Design review of the part shown in the three views and the two pictorial views. Dimensions are in mm from the part's minimum x, y and z. Round coordinates to 2 decimals unless told otherwise and drop trailing zeros. Order: outer loops, then holes, each group sorted by start corner. A loop starts at its lowest first (then second) coordinate and runs counter-clockwise, first axis right, second up.
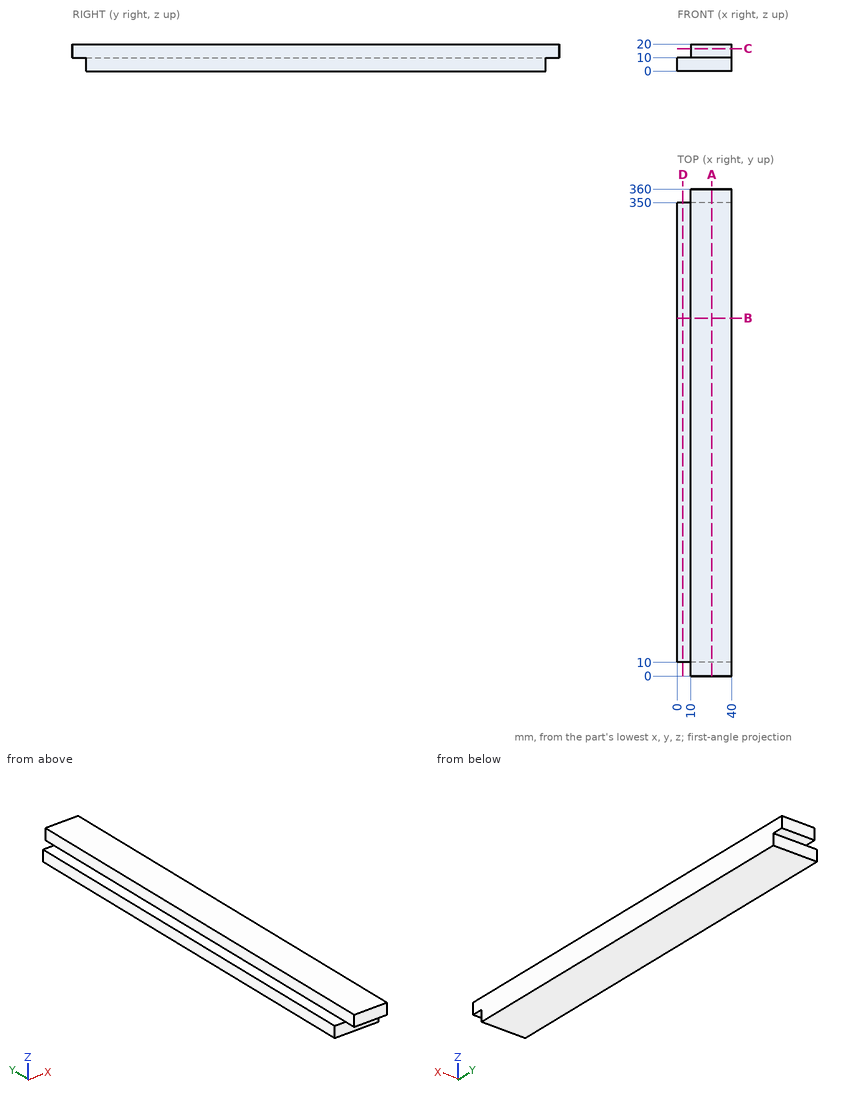
(1) To check wall thickness, follow probe 1 along Y at (x, z) = (14.5, 7.5); probe 2 along X at (y, z) = (243, 15); probe 3 along Z at (x, y) = (7, 153). State the ranges of each line that lie inside material, in increasing order.
Data:
probe 1: y = 10 to 350
probe 2: x = 10 to 40
probe 3: z = 0 to 10
(2) Consider section A-A (x = 25.5). Write out the cut boundary in (y, z), and give its area (3 significant figures).
Data:
outline: (0, 10) - (10, 10) - (10, 0) - (350, 0) - (350, 10) - (360, 10) - (360, 20) - (0, 20) - close
area: 7,000 mm2
(3) Consider section D-D (x = 4). Write out the cut boundary in (y, z), and give its area (3 significant figures).
Data:
outline: (10, 0) - (350, 0) - (350, 10) - (10, 10) - close
area: 3,400 mm2
(4) Consider section B-B (y = 264.5). Write out the cut boundary in (x, z).
Data:
outline: (0, 0) - (40, 0) - (40, 20) - (10, 20) - (10, 10) - (0, 10) - close
(5) Consider section C-C (z = 16.5). Write out the cut boundary in (x, y).
Data:
outline: (10, 0) - (40, 0) - (40, 360) - (10, 360) - close
(6) Insertion check: pin 1 (8 mm diameter, centred on y = 203.5, z = 16.5, fed in from -X); pin 2 (3 mm diameter, centred on x = 2.5, y = 147.5, fed in from +Z); pin 3 (5 mm diameter, centred on x = 18.5, y = 357.5, fed in from -Z). Each pin has a flat end and moves straight along its axis. Give the tip position at first contact, or say it passes through.
Data:
pin 1: stops at x = 10
pin 2: stops at z = 10
pin 3: stops at z = 10
